Here's how the part is built. I have some questions about the finished solid (model axes, mm). A direction names the side the tool comes from. Give positions to 0.01 mm unless a question says otherwise; leave off trailing zeros. Write each loop counter-clockwise with the first axis right and the second up, starting at its lowest first coordinate (ties: lowest second). Pieces come first, ordered by that corner, then holes. Notation, with made-up numbers: (35, -13.75) -> (75, -13.75) arc R18 cw to (75, -6.75) -> close; hole circle Ø8 at (73.25, 26.25). An arc over 180 degrees is marked (long way). Use one line per item in the form item = value.
```python
from build123d import *

# Parameters (mm, degrees)
SKETCH1_R               = 2.54
BOSS_EXTRUDE1_DEPTH     = 18.1991
SKETCH2_W               = 63.5
SKETCH2_H               = 22.225
BOSS_EXTRUDE2_DEPTH     = 9.271
CUT_EXTRUDE1_DEPTH      = 61.187575184
CUT_EXTRUDE1_DEPTH_BACK = 61.187575184
SKETCH3_R               = 1.5875


with BuildPart() as part:
    # Sketch1 → Boss-Extrude1 (new, symmetric)
    with BuildSketch(Plane.XY):
        Circle(SKETCH1_R)
    extrude(amount=BOSS_EXTRUDE1_DEPTH, both=True)

    # Sketch2 → Boss-Extrude2 (add, symmetric)
    with BuildSketch(Plane.XY):
        with Locations((20.6375, 0)):
            Rectangle(SKETCH2_W, SKETCH2_H)
    extrude(amount=BOSS_EXTRUDE2_DEPTH, both=True)

    # Sketch3 → Cut-Extrude1 (cut, two sides: drawn at the far end of the back side and taken through both)
    with BuildSketch(Plane.XY.offset(9.271).offset(-CUT_EXTRUDE1_DEPTH_BACK)):
        with Locations((19.05, -8.73125)):
            Circle(SKETCH3_R)
        with Locations((19.05, 8.73125)):
            Circle(SKETCH3_R)
    extrude(amount=CUT_EXTRUDE1_DEPTH + CUT_EXTRUDE1_DEPTH_BACK, mode=Mode.SUBTRACT)


solid = part.part
```
Q1. I want a section at D-D, the plane z = -11. Write out the boundary of the cut face in (x, y), and give its area (3 significant figures).
Result set:
outline = circle Ø5.08 at (0, 0)
area = 20.3 mm2
Q2. Which directions (+Z, -Z, +X, -X, +Y, -Y) give clear straight access to the entire face, cutting with the end or side of a thin tool? Please do faces 1 (the face through (17.464, -8.661, -0.13)), 2 (the face through (-0.33, 2.52, -13.67)).
Result set:
face_1 = +Z, -Z
face_2 = -Z
Q3. I want a section at C-C, the plane x = 0. Write out the boundary of the cut face in (y, z).
Result set:
outline = (-11.11, -9.27) -> (-2.54, -9.27) -> (-2.54, -18.2) -> (2.54, -18.2) -> (2.54, -9.27) -> (11.11, -9.27) -> (11.11, 9.27) -> (2.54, 9.27) -> (2.54, 18.2) -> (-2.54, 18.2) -> (-2.54, 9.27) -> (-11.11, 9.27) -> close
Q4. I want a section at B-B, the plane y = 0. Write out the boundary of the cut face in (x, z), and give its area (3 significant figures).
Result set:
outline = (-11.11, -9.27) -> (-2.54, -9.27) -> (-2.54, -18.2) -> (2.54, -18.2) -> (2.54, -9.27) -> (52.39, -9.27) -> (52.39, 9.27) -> (2.54, 9.27) -> (2.54, 18.2) -> (-2.54, 18.2) -> (-2.54, 9.27) -> (-11.11, 9.27) -> close
area = 1,270 mm2
Q5. If we mould it in two halves opening along Y, with no side actions, what happens to faces 3 (the face through (20, 11.112, 0)), 4 (the face through (17.88, 9.804, -0.13)), 5 (the face through (-0.33, 2.52, 13.8))? For each: +Y half, -Y half, draft (parallel to the pull), parting line (faces both ways), or undercut.
Result set:
face_3 = +Y half
face_4 = undercut
face_5 = parting line
Q6. I want a section at A-A, the plane x = 19.05. Write out the boundary of the cut face in (y, z), and give its area (3 significant figures).
Result set:
outline = (-11.11, -9.27) -> (-10.32, -9.27) -> (-10.32, 9.27) -> (-11.11, 9.27) -> close; (-7.14, -9.27) -> (7.14, -9.27) -> (7.14, 9.27) -> (-7.14, 9.27) -> close; (10.32, -9.27) -> (11.11, -9.27) -> (11.11, 9.27) -> (10.32, 9.27) -> close
area = 294 mm2
Q7. If I drill on line 1 along Y through (x, z) = (19.05, -0.25); line 2 along Z through (x, y) = (15.5, -3.5); line 3 along X through (y, z) = (8.5, -5.5), over which ranges is the centre line in solid material (lowest first)? Write a range as from..to.
Result set:
line_1 = -11.11..-10.32, -7.14..7.14, 10.32..11.11
line_2 = -9.27..9.27
line_3 = -11.11..17.48, 20.62..52.39
Q8. Will these pins go through, and if not, where does the flat tip stop? pin 1 Ø6 at (y, z) = (-4, 12) entering from +X; pin 2 Ø1.9 at (x, y) = (19.05, -8.73) entering from -Z; pin 3 Ø6 at (x, y) = (-2.5, 5.5) entering from -Z; pin 4 Ø1 at (x, y) = (37.5, -6.5) entering from +Z.
Result set:
pin_1 = 52.39
pin_2 = through
pin_3 = -9.27
pin_4 = 9.27
